Build history of the part. All positions in model axes, mm. A direction names the side the tool comes from. Coordinates: 2 decimals unless noted, no trailing zeros. Order: outer loops, then holes, each group sorted by start corner. A loop starts at its lowest first (then second) coordinate and runs counter-clockwise, first axis right, second up. Notation, with made-up numbers: (-14, 17.5) -> (1, 17.5) arc R10 cw to (1, 33.5) -> close; hole circle Ø7 at (51, 65.25). An arc over 180 degrees is marked (long way). Write each question's results on one line, items separated by ' | '.
from build123d import *

# Parameters (mm, degrees)
SKETCH1_R           = 27
SKETCH1_R_2         = 1.750000056
SKETCH1_R_3         = 1.75
BOSS_EXTRUDE1_DEPTH = 12.5
SKETCH6_R           = 35
CUT_EXTRUDE3_DEPTH  = 7.5
SKETCH7_R           = 33.747750153
SKETCH7_R_2         = 27
BOSS_EXTRUDE4_DEPTH = 14.125838812
SKETCH8_R           = 33.747750153
SKETCH8_R_2         = 16
BOSS_EXTRUDE5_DEPTH = 2.54
SKETCH9_R           = 2.499999953
CUT_EXTRUDE4_DEPTH  = 5


with BuildPart() as part:
    # Sketch1 → Boss-Extrude1 (new body)
    with BuildSketch(Plane(origin=(0, 0, 0), x_dir=(0, 0, -1), z_dir=(1, 0, 0))):
        with BuildLine():
            Line((46.5, 0), (46.5, -46.5))
            Line((46.5, -46.5), (-46.5, -46.5))
            Line((-46.5, -46.5), (-46.5, 0))
            ThreePointArc((-46.5, 0), (0, 46.5), (46.5, 0))
        make_face()
        Circle(SKETCH1_R, mode=Mode.SUBTRACT)
        with Locations((15.5, 26.846787517)):
            Circle(SKETCH1_R_2, mode=Mode.SUBTRACT)
        with Locations((0, 31)):
            Circle(SKETCH1_R_2, mode=Mode.SUBTRACT)
        with Locations((-15.5, 26.846787517)):
            Circle(SKETCH1_R_2, mode=Mode.SUBTRACT)
        with Locations((-31, 0)):
            Circle(SKETCH1_R_2, mode=Mode.SUBTRACT)
        with Locations((-26.846787517, -15.5)):
            Circle(SKETCH1_R_2, mode=Mode.SUBTRACT)
        with Locations((-15.5, -26.846787517)):
            Circle(SKETCH1_R_2, mode=Mode.SUBTRACT)
        with Locations((0, -31)):
            Circle(SKETCH1_R_2, mode=Mode.SUBTRACT)
        with Locations((15.5, -26.846787517)):
            Circle(SKETCH1_R_2, mode=Mode.SUBTRACT)
        with Locations((26.846787517, -15.5)):
            Circle(SKETCH1_R_2, mode=Mode.SUBTRACT)
        with Locations((31, 0)):
            Circle(SKETCH1_R_2, mode=Mode.SUBTRACT)
        with Locations((26.846787517, 15.5)):
            Circle(SKETCH1_R_2, mode=Mode.SUBTRACT)
        with Locations((-26.846787517, 15.5)):
            Circle(SKETCH1_R_3, mode=Mode.SUBTRACT)
        with Locations((0, 40)):
            Circle(SKETCH1_R_3, mode=Mode.SUBTRACT)
        with Locations((25.711504387, 30.641777725)):
            Circle(SKETCH1_R_3, mode=Mode.SUBTRACT)
        with Locations((39.39231012, 6.945927107)):
            Circle(SKETCH1_R_3, mode=Mode.SUBTRACT)
        with Locations((34.641016151, -20)):
            Circle(SKETCH1_R_3, mode=Mode.SUBTRACT)
        with Locations((13.680805733, -37.587704831)):
            Circle(SKETCH1_R_3, mode=Mode.SUBTRACT)
        with Locations((-13.680805733, -37.587704831)):
            Circle(SKETCH1_R_3, mode=Mode.SUBTRACT)
        with Locations((-34.641016151, -20)):
            Circle(SKETCH1_R_3, mode=Mode.SUBTRACT)
        with Locations((-39.39231012, 6.945927107)):
            Circle(SKETCH1_R_3, mode=Mode.SUBTRACT)
        with Locations((-25.711504387, 30.641777725)):
            Circle(SKETCH1_R_3, mode=Mode.SUBTRACT)
    extrude(amount=BOSS_EXTRUDE1_DEPTH)

    # Sketch6 → Cut-Extrude3 (cut)
    with BuildSketch(Plane.ZY):
        Circle(SKETCH6_R)
    extrude(amount=-CUT_EXTRUDE3_DEPTH, mode=Mode.SUBTRACT)

    # Sketch7 → Boss-Extrude4 (add)
    with BuildSketch(Plane(origin=(12.5, 0, 0), x_dir=(0, 0, -1), z_dir=(1, 0, 0))):
        Circle(SKETCH7_R)
        with Locations(Location((0, 0, 0), (0, 0, 180))):
            Circle(SKETCH7_R_2, mode=Mode.SUBTRACT)
    extrude(amount=BOSS_EXTRUDE4_DEPTH)

    # Sketch8 → Boss-Extrude5 (add)
    with BuildSketch(Plane(origin=(26.625838812, 0, 0), x_dir=(0, 0, -1), z_dir=(1, 0, 0))):
        Circle(SKETCH8_R)
        Circle(SKETCH8_R_2, mode=Mode.SUBTRACT)
    extrude(amount=BOSS_EXTRUDE5_DEPTH)

    # Sketch9 → Cut-Extrude4 (cut)
    with BuildSketch(Plane.XZ.offset(46.5)):
        with Locations(Location((6.25, 37.338000036, 0), (0, 0, 270))):
            Circle(SKETCH9_R)
        with Locations(Location((6.25, 24.892000036, 0), (0, 0, 270))):
            Circle(SKETCH9_R)
        with Locations(Location((6.25, 12.446000036, 0), (0, 0, 270))):
            Circle(SKETCH9_R)
        with Locations(Location((6.25, 3.6e-08, 0), (0, 0, 270))):
            Circle(SKETCH9_R)
        with Locations(Location((6.25, -12.445999964, 0), (0, 0, 270))):
            Circle(SKETCH9_R)
        with Locations(Location((6.25, -24.891999964, 0), (0, 0, 270))):
            Circle(SKETCH9_R)
        with Locations(Location((6.25, -37.337999964, 0), (0, 0, 270))):
            Circle(SKETCH9_R)
    extrude(amount=-CUT_EXTRUDE4_DEPTH, mode=Mode.SUBTRACT)


solid = part.part
Item 1: Slice it at A-A, the plane y = -20. List the corners of the cut face in (x, z), and give its area (3 significant figures).
Answer:
outline: (0, -46.5) -> (12.5, -46.5) -> (12.5, -36.39) -> (0, -36.39) -> close; (0, -32.89) -> (12.5, -32.89) -> (12.5, -27.18) -> (29.17, -27.18) -> (29.17, 27.18) -> (12.5, 27.18) -> (12.5, 32.89) -> (0, 32.89) -> (0, 28.72) -> (7.5, 28.72) -> (7.5, 18.14) -> (26.63, 18.14) -> (26.63, -18.14) -> (7.5, -18.14) -> (7.5, -28.72) -> (0, -28.72) -> close; (0, 36.39) -> (12.5, 36.39) -> (12.5, 46.5) -> (0, 46.5) -> close | area: 856 mm^2
Item 2: Slice it at B-B, the plane x = 22. List the corners of the cut face in (y, z), and give its area (3 significant figures).
Answer:
outline: circle Ø67.5 at (0, 0); hole circle Ø54 at (0, 0) | area: 1,290 mm^2
Item 3: Slice it at C-C, the plane y = 40. List the corners of the cut face in (x, z).
Answer:
outline: (0, -23.71) -> (12.5, -23.71) -> (12.5, -1.75) -> (0, -1.75) -> close; (0, 1.75) -> (12.5, 1.75) -> (12.5, 23.71) -> (0, 23.71) -> close
Item 4: Tool access for faces 1 (the cylindrical face through (6.162, -18.524, 33.7)), 2 (the flat face through (12.5, 27, 16)), 3 (the flat face through (6, -41.5, 25)): list every direction of +Z, -Z, +X, -X, +Y, -Y with a clear straight run to the whole face (end or side of a thin tool).
Answer:
face 1: +X, -X | face 2: -X | face 3: -Y
Item 5: Pull direction Z, two halves, no side cores. Call faces 4 (the cylindrical face through (9.965, 32.735, 0.228)), 5 (the flat face through (12.5, -30, 20)): released by +Z, released by -Z, zero draft, split by the parting line, or undercut.
Answer:
face 4: undercut | face 5: zero draft
Item 6: Pin check, flat tips, straight feed: pin 1 (1.5 mm diameter, centred on x = 5.5, z = 12, fed in from -Y); pin 2 (1 mm diameter, centred on x = 22.5, z = 18.5, fed in from -Y); pin 3 (1.5 mm diameter, centred on y = -35.5, z = -27, fed in from +X); pin 4 (5.5 mm diameter, centred on y = -37.59, z = -13.68, fed in from -X). Stop position of each tip, or through.
Answer:
pin 1: stops at y = -41.5 | pin 2: stops at y = -28.55 | pin 3: stops at x = 12.5 | pin 4: stops at x = 0
Item 7: Drill centre lines: line 1 (Y direction, x = 8, z = 0); line 2 (Y direction, x = 17, z = 0); line 3 (X direction, y = 3.5, z = 39). Where is each one in solid material? Low to high. Write a range as from..to.
Answer:
line 1: y = -41.5..-32.75, -29.25..-27, 27..29.25, 32.75..38.25, 41.75..46.5 | line 2: y = -33.75..-27, 27..33.75 | line 3: x = 0..12.5
